from build123d import *

# Parameters (mm, degrees)
PAD_DEPTH = 20
FILLET_R  = 3


with BuildPart() as part:
    # Sketch → Pad (new body)
    with BuildSketch(Plane.XY):
        Polygon((9.1, 0), (9.1, -40), (19.1, -40), (19.1, 10), (-19.1, 10), (-19.1, -50), (-49.1, -50), (-49.1, 10), (-59.1, 10), (-59.1, -60), (-9.1, -60), (-9.1, 0), align=None)
    extrude(amount=PAD_DEPTH)

    # Fillet
    fillet_edges = [part.edges().sort_by_distance(p)[0] for p in [
        (9.1, 0, 10),
        (9.1, -40, 10),
        (9.1, -20, 0),
        (9.1, -20, 20),
        (19.1, -40, 10),
        (14.1, -40, 0),
        (14.1, -40, 20),
        (19.1, 10, 10),
        (19.1, -15, 0),
        (19.1, -15, 20),
        (-19.1, 10, 10),
        (0, 10, 0),
        (0, 10, 20),
        (-19.1, -50, 10),
        (-19.1, -20, 0),
        (-19.1, -20, 20),
        (-49.1, -50, 10),
        (-34.1, -50, 0),
        (-34.1, -50, 20),
        (-49.1, 10, 10),
        (-49.1, -20, 0),
        (-49.1, -20, 20),
        (-59.1, 10, 10),
        (-54.1, 10, 0),
        (-54.1, 10, 20),
        (-59.1, -60, 10),
        (-59.1, -25, 0),
        (-59.1, -25, 20),
        (-9.1, -60, 10),
        (-34.1, -60, 0),
        (-34.1, -60, 20),
        (-9.1, 0, 10),
        (-9.1, -30, 0),
        (-9.1, -30, 20),
        (0, 0, 0),
        (0, 0, 20),
    ]]
    fillet(fillet_edges, radius=FILLET_R)


solid = part.part
The listing builds one solid part. Answer for the finished solid, in the listing's coordinates (mm). A direction names the side the tool comes from. Coordinates: 2 decimals unless noted, no trailing zeros. Loops run counter-clockwise (first coordinate to the right, second up) from the corner with the lowest first, then second, coordinate; pieces in that order, holes last. Notation, with made-up numbers: M -26,-25 L 26,-25 A17 cw 26,-6 Z; hole C 34.5,54 d10. An arc over 180 degrees is marked long. Answer in a Markdown table with one row per item.
1) Determine the mould class of faces 6 (the cylindrical face through (-58.24, -25.45, 0.9)), 7 (the cylindrical face through (14.13, -39.14, 19.1)), 8 (the cylindrical face through (18.24, -14.69, 19.1)), 9 (the cylindrical face through (-49.96, 9.1, 10.1)) for opening direction X: released by +X, released by -X, zero draft, split by the parting line, or undercut.
Answers below:
| item | result |
|---|---|
| face 6 | released by -X |
| face 7 | zero draft |
| face 8 | released by +X |
| face 9 | undercut |
2) Find the intervals of material crossed by probe 1 along X at (y, z) = (-17.5, 11.75); probe 2 along X at (y, z) = (3.5, 10.25); probe 3 along X at (y, z) = (-43.5, 10.5), in increasing order.
Answers below:
| item | result |
|---|---|
| probe 1 | -59.1 to -49.1, -19.1 to -9.1, 9.1 to 19.1 |
| probe 2 | -59.1 to -49.1, -19.1 to 19.1 |
| probe 3 | -59.1 to -49.1, -19.1 to -9.1 |
3) Find section C-C (z = 15.75). Determine the outline of the cut face in (x, y), then the cut area to 3 significant figures.
Answers below:
| item | result |
|---|---|
| outline | M -59.1,-57 A3 ccw -56.1,-60 L -12.1,-60 A3 ccw -9.1,-57 L -9.1,-3 A3 cw -6.1,0 L 6.1,0 A3 cw 9.1,-3 L 9.1,-37 A3 ccw 12.1,-40 L 16.1,-40 A3 ccw 19.1,-37 L 19.1,7 A3 ccw 16.1,10 L -16.1,10 A3 ccw -19.1,7 L -19.1,-47 A3 cw -22.1,-50 L -46.1,-50 A3 cw -49.1,-47 L -49.1,7 A3 ccw -52.1,10 L -56.1,10 A3 ccw -59.1,7 Z |
| area | 2,370 mm^2 |
4) Given pin 1 (4 mm diameter, centred on x = -29, z = 11.5, fed in from +Y); pin 2 (3 mm diameter, centred on x = 3.5, z = 13.5, fed in from -Y); pin 3 (10 mm diameter, centred on y = -50.5, z = 3.5, fed in from +X), each flat-ended and moving along its own axis, determine where each tip first touches the part or whether it passes through.
Answers below:
| item | result |
|---|---|
| pin 1 | y = -50 |
| pin 2 | y = 0 |
| pin 3 | x = -9.1 |
5) Which of the six approach directions +Z, -Z, +X, -X, +Y, -Y give full straight-line access (tool end or side, diameter ignored) to faces 1 (the cylindrical face through (-18.24, -20.38, 0.9)), 2 (the cylindrical face through (-8.24, -0.9, 10.1)), 3 (the cylindrical face through (-18.24, -20.38, 19.1)), 4 (the cylindrical face through (14.13, -39.14, 0.9)), 5 (the cylindrical face through (-9.96, -29.62, 19.1))?
Answers below:
| item | result |
|---|---|
| face 1 | -Z, +Y |
| face 2 | +Z, -Z, -Y |
| face 3 | +Z, +Y |
| face 4 | -Z, +X, -Y |
| face 5 | +Z, -Y |
6) Find section B-B (x = -4.5). Determine the outline of the cut face in (y, z).
Answers below:
| item | result |
|---|---|
| outline | M 0,3 A3 ccw 3,0 L 7,0 A3 ccw 10,3 L 10,17 A3 ccw 7,20 L 3,20 A3 ccw 0,17 Z |
7) Find section A-A (y = -35). Determine the outline of the cut face in (x, z).
Answers below:
| item | result |
|---|---|
| outline | M -59.1,3 A3 ccw -56.1,0 L -52.1,0 A3 ccw -49.1,3 L -49.1,17 A3 ccw -52.1,20 L -56.1,20 A3 ccw -59.1,17 Z; M -19.1,3 A3 ccw -16.1,0 L -12.1,0 A3 ccw -9.1,3 L -9.1,17 A3 ccw -12.1,20 L -16.1,20 A3 ccw -19.1,17 Z; M 9.1,3 A3 ccw 12.1,0 L 16.1,0 A3 ccw 19.1,3 L 19.1,17 A3 ccw 16.1,20 L 12.1,20 A3 ccw 9.1,17 Z |
